Work out the finished part from the listing and answer in its coordinate system (mm). A direction names the side the tool comes from. Round coordinates to 2 decimals unless told otherwise and drop trailing zeros. Loops run counter-clockwise (first coordinate to the right, second up) from the corner with the lowest first, then second, coordinate; pieces in that order, holes last.
```python
from build123d import *

# Parameters (mm, degrees)
BOSS_1_DEPTH  = 5.6
BOSS_2_DEPTH  = 4.95
CUT_3_DEPTH   = 1.1
CUT_4_DEPTH   = 1.1
CUT_5_DEPTH   = 1.1
CUT_6_DEPTH   = 1.1
CUT_7_DEPTH   = 1.7
CUT_8_DEPTH   = 1.7
CUT_9_DEPTH   = 1.9
CUT_10_DEPTH  = 2.9
S_HOLE11_R    = 1.2
HOLE_11_DEPTH = 8.8
S_HOLE12_R    = 2.3
HOLE_12_DEPTH = 3.1
S_HOLE13_R    = 1.2
HOLE_13_DEPTH = 8.8
S_HOLE14_R    = 2.3
HOLE_14_DEPTH = 3.1
S_HOLE15_R    = 1.2
HOLE_15_DEPTH = 8.8
S_HOLE16_R    = 2.3
HOLE_16_DEPTH = 3.1
S_HOLE17_R    = 1.2
HOLE_17_DEPTH = 8.8
S_HOLE18_R    = 2.3
HOLE_18_DEPTH = 3.1
S_HOLE19_R    = 1.2
HOLE_19_DEPTH = 8.8
S_HOLE20_R    = 2.3
HOLE_20_DEPTH = 3.1


with BuildPart() as part:
    # S_prism1 → Boss_1 (new body)
    with BuildSketch(Plane.XY.offset(24.6)):
        with BuildLine():
            Line((-14.912987345, 21.297953152), (-11.242098152, 16.055380068))
            ThreePointArc((-11.242098152, 16.055380068), (15.014471085, 12.59863715), (13.859292911, -13.859292911))
            Line((13.859292911, -13.859292911), (18.384776311, -18.384776311))
            ThreePointArc((18.384776311, -18.384776311), (19.917155521, 16.712477852), (-14.912987345, 21.297953152))
        make_face()
    extrude(amount=BOSS_1_DEPTH)

    # S_prism2 → Boss_2 (add)
    with BuildSketch(Plane.XY.offset(21.6)):
        with BuildLine():
            Line((-13.68454789, 19.594467307), (-8.932173518, 12.789694142))
            ThreePointArc((-8.932173518, 12.789694142), (11.950293313, 10.027486711), (11.044334296, -11.017380812))
            Line((11.044334296, -11.017380812), (16.920486517, -16.879192399))
            ThreePointArc((16.920486517, -16.879192399), (18.308462191, 15.362623872), (-13.68454789, 19.594467307))
        make_face()
    extrude(amount=BOSS_2_DEPTH)

    # S_pcut3 → Cut_3 (cut)
    with BuildSketch(Plane.XY.offset(24.5)):
        with BuildLine():
            Line((-15.39997361, 21.196245253), (-14.04806753, 19.335506166))
            ThreePointArc((-14.04806753, 19.335506166), (18.308462191, 15.362623872), (16.602335054, -17.192221228))
            Line((16.602335054, -17.192221228), (18.200049306, -18.846702769))
            ThreePointArc((18.200049306, -18.846702769), (20.07036441, 16.841035374), (-15.39997361, 21.196245253))
        make_face()
    extrude(amount=CUT_3_DEPTH, mode=Mode.SUBTRACT)

    # S_pcut4 → Cut_4 (cut)
    with BuildSketch(Plane.XY.offset(21.5)):
        with BuildLine():
            Line((-9.992349289, 13.753288904), (-9.110671411, 12.539763413))
            ThreePointArc((-9.110671411, 12.539763413), (11.873688868, 9.96320795), (10.767204742, -11.149766905))
            Line((10.767204742, -11.149766905), (11.809192298, -12.228776606))
            ThreePointArc((11.809192298, -12.228776606), (13.022755533, 10.927389365), (-9.992349289, 13.753288904))
        make_face()
    extrude(amount=CUT_4_DEPTH, mode=Mode.SUBTRACT)

    # S_pcut5 → Cut_5 (cut)
    with BuildSketch(Plane.XY.offset(21.5)):
        with BuildLine():
            Line((-10.697691592, 14.724109298), (-9.110671411, 12.539763413))
            ThreePointArc((-9.110671411, 12.539763413), (-0.811207322, 15.478757789), (7.75, 13.423393759))
            Line((7.75, 13.423393759), (9.1, 15.761662349))
            ThreePointArc((9.1, 15.761662349), (-0.952514404, 18.175057533), (-10.697691592, 14.724109298))
        make_face()
    extrude(amount=CUT_5_DEPTH, mode=Mode.SUBTRACT)

    # S_pcut6 → Cut_6 (cut)
    with BuildSketch(Plane.XY.offset(21.5)):
        with BuildLine():
            Line((18.545775865, -4.969325666), (14.971850307, -4.011695199))
            ThreePointArc((14.971850307, -4.011695199), (13.355251987, -7.866844626), (10.767204742, -11.149766905))
            Line((10.767204742, -11.149766905), (13.337440713, -13.811324167))
            ThreePointArc((13.337440713, -13.811324167), (16.54327988, -9.744736569), (18.545775865, -4.969325666))
        make_face()
    extrude(amount=CUT_6_DEPTH, mode=Mode.SUBTRACT)

    # S_pcut7 → Cut_7 (cut)
    with BuildSketch(Plane.XY.offset(21.5)):
        with BuildLine():
            Line((25.307256649, -6.781058982), (19.608294274, -5.254026616))
            ThreePointArc((19.608294274, -5.254026616), (17.491071957, -10.303028768), (14.10156492, -14.602597947))
            Line((14.10156492, -14.602597947), (18.200049306, -18.846702769))
            ThreePointArc((18.200049306, -18.846702769), (22.574684004, -13.29750511), (25.307256649, -6.781058982))
        make_face()
    extrude(amount=CUT_7_DEPTH, mode=Mode.SUBTRACT)

    # S_pcut8 → Cut_8 (cut)
    with BuildSketch(Plane.XY.offset(21.5)):
        with BuildLine():
            Line((-15.39997361, 21.196245253), (-11.932040622, 16.423044986))
            ThreePointArc((-11.932040622, 16.423044986), (-1.062419912, 20.272179556), (10.15, 17.580315697))
            Line((10.15, 17.580315697), (13.1, 22.689865579))
            ThreePointArc((13.1, 22.689865579), (-1.371202054, 26.164093811), (-15.39997361, 21.196245253))
        make_face()
    extrude(amount=CUT_8_DEPTH, mode=Mode.SUBTRACT)

    # S_pcut9 → Cut_9 (cut)
    with BuildSketch(Plane.XY.offset(21.5)):
        with BuildLine():
            Line((-15.39997361, 21.196245253), (-11.932040622, 16.423044986))
            ThreePointArc((-11.932040622, 16.423044986), (-8.739375265, 18.322481272), (-5.254026616, 19.608294274))
            Line((-5.254026616, 19.608294274), (-6.781058982, 25.307256649))
            ThreePointArc((-6.781058982, 25.307256649), (-11.279390736, 23.64773445), (-15.39997361, 21.196245253))
        make_face()
    extrude(amount=CUT_9_DEPTH, mode=Mode.SUBTRACT)

    # S_pcut10 → Cut_10 (cut)
    with BuildSketch(Plane.XY.offset(21.5)):
        with BuildLine():
            Line((-15.39997361, 21.196245253), (-12.519825874, 17.23206198))
            ThreePointArc((-12.519825874, 17.23206198), (-10.326444911, 18.629399762), (-7.97912044, 19.749016102))
            Line((-7.97912044, 19.749016102), (-9.814692747, 24.29221699))
            ThreePointArc((-9.814692747, 24.29221699), (-12.70201205, 22.915036327), (-15.39997361, 21.196245253))
        make_face()
    extrude(amount=CUT_10_DEPTH, mode=Mode.SUBTRACT)

    # S_hole11 → Hole_11 (cut)
    with BuildSketch(Plane.XY.offset(21.5)):
        with Locations((18.021344974, -12.6186816)):
            Circle(S_HOLE11_R)
    extrude(amount=HOLE_11_DEPTH, mode=Mode.SUBTRACT)

    # S_hole12 → Hole_12 (cut)
    with BuildSketch(Plane.XY.offset(21.5)):
        with Locations((18.021344974, -12.6186816)):
            Circle(S_HOLE12_R)
    extrude(amount=HOLE_12_DEPTH, mode=Mode.SUBTRACT)

    # S_hole13 → Hole_13 (cut)
    with BuildSketch(Plane.XY.offset(21.5)):
        with Locations((21.916283358, 1.91742634)):
            Circle(S_HOLE13_R)
    extrude(amount=HOLE_13_DEPTH, mode=Mode.SUBTRACT)

    # S_hole14 → Hole_14 (cut)
    with BuildSketch(Plane.XY.offset(21.5)):
        with Locations((21.916283358, 1.91742634)):
            Circle(S_HOLE14_R)
    extrude(amount=HOLE_14_DEPTH, mode=Mode.SUBTRACT)

    # S_hole15 → Hole_15 (cut)
    with BuildSketch(Plane.XY.offset(21.5)):
        with Locations((15.556349186, 15.556349186)):
            Circle(S_HOLE15_R)
    extrude(amount=HOLE_15_DEPTH, mode=Mode.SUBTRACT)

    # S_hole16 → Hole_16 (cut)
    with BuildSketch(Plane.XY.offset(21.5)):
        with Locations((15.556349186, 15.556349186)):
            Circle(S_HOLE16_R)
    extrude(amount=HOLE_16_DEPTH, mode=Mode.SUBTRACT)

    # S_hole17 → Hole_17 (cut)
    with BuildSketch(Plane.XY.offset(21.5)):
        with Locations((1.91742634, 21.916283358)):
            Circle(S_HOLE17_R)
    extrude(amount=HOLE_17_DEPTH, mode=Mode.SUBTRACT)

    # S_hole18 → Hole_18 (cut)
    with BuildSketch(Plane.XY.offset(21.5)):
        with Locations((1.91742634, 21.916283358)):
            Circle(S_HOLE18_R)
    extrude(amount=HOLE_18_DEPTH, mode=Mode.SUBTRACT)

    # S_hole19 → Hole_19 (cut)
    with BuildSketch(Plane.XY.offset(21.5)):
        with Locations(Location((-9.297601758, 19.938771315, 0), (0, 0, 241.964907162))):
            Circle(S_HOLE19_R)
    extrude(amount=HOLE_19_DEPTH, mode=Mode.SUBTRACT)

    # S_hole20 → Hole_20 (cut)
    with BuildSketch(Plane.XY.offset(21.5)):
        with Locations((-9.297601758, 19.938771315)):
            Circle(S_HOLE20_R)
    extrude(amount=HOLE_20_DEPTH, mode=Mode.SUBTRACT)


solid = part.part
```
1. Consider probe 1 along X at (y, z) = (22, 28.75); probe 2 along Z at (x, y) = (22, 4); probe 3 along X at (y, z) = (13.5, 25.25). Determine where each line is inside the solid, lowest interval first.
Answer key:
probe 1: x = -13.86 to 0.72, 3.11 to 13.86
probe 2: z = 24.6 to 30.2
probe 3: x = -9.43 to -7.82, 7.82 to 19.72
2. Determine the mould class of faces 6 (the face through (-0.64, 18.19, 22.09)), 7 (the face through (16.6, -9.65, 22.09)), 8 (the face through (18.624, 14.979, 24.016)) for opening direction X: +X half, -X half, draft (parallel to the pull), parting line (faces both ways), or undercut.
Answer key:
face 6: undercut
face 7: -X half
face 8: parting line
3. Find section B-B (x = 6). Write down the section's boundary in (y, z), then the cut area to 3 significant figures.
Answer key:
outline: (14.4, 22.6) - (17.18, 22.6) - (17.18, 21.6) - (19.39, 21.6) - (19.39, 23.2) - (23.13, 23.2) - (23.13, 25.6) - (25.3, 25.6) - (25.3, 30.2) - (18.66, 30.2) - (18.66, 26.55) - (14.4, 26.55) - close
area: 60.8 mm2
4. Given pin 1 (2 mm diameter, centred on y = 20, z = 23, fed in from +X); pin 2 (2 mm diameter, centred on x = 14.5, z = 23.5, fed in from +Y); pin 3 (5 mm diameter, centred on x = -9, z = 28.5, fed in from +Y); pin 4 (14.5 mm diameter, centred on x = 0, y = 7.5, fed in from -Z), each flat-ended and moving along its own axis, determine where each tip first touches the part or whether it passes through.
Answer key:
pin 1: stops at x = 14.5
pin 2: stops at y = 19.72
pin 3: stops at y = 25.17
pin 4: passes through
5. Which of the six approach directions +Z, -Z, +X, -X, +Y, -Y give full straight-line access (tool end or side, diameter ignored) to faces 1 (the face through (11.04, 19.12, 22.39)), 2 (the face through (13, 9, 22.6)), 3 (the face through (15.08, -13.59, 22.39)), 4 (the face through (18.7, -7.9, 22.4)), 5 (the face through (-11.568, 17.885, 23.893))?
Answer key:
face 1: -Z, +Y
face 2: -Z
face 3: -Z, +X, -Y
face 4: -Z, -Y
face 5: -Z, -X, +Y
6. Find section C-C (y = 7). Write down the section's boundary in (x, z).
Answer key:
outline: (13.94, 22.6) - (15.49, 22.6) - (15.49, 21.6) - (22.85, 21.6) - (22.85, 25.6) - (25.04, 25.6) - (25.04, 30.2) - (18.31, 30.2) - (18.31, 26.55) - (13.94, 26.55) - close
7. Find section D-D (y = 12). Write down the section's boundary in (x, z), then the cut area to 3 significant figures.
Answer key:
outline: (9.97, 22.6) - (12.04, 22.6) - (12.04, 21.6) - (20.67, 21.6) - (20.67, 25.6) - (23.07, 25.6) - (23.07, 30.2) - (15.5, 30.2) - (15.5, 26.55) - (9.97, 26.55) - close
area: 80.8 mm2
8. Find section A-A (z = 28.25). Write down the section's boundary in (x, y).
Answer key:
outline: (-14.91, 21.3) - (-11.24, 16.06) arc R19.6 cw to (13.86, -13.86) - (18.38, -18.38) arc R26 ccw to start; hole circle Ø2.4 at (-9.3, 19.94); hole circle Ø2.4 at (1.92, 21.92); hole circle Ø2.4 at (15.56, 15.56); hole circle Ø2.4 at (18.02, -12.62); hole circle Ø2.4 at (21.92, 1.92)
